Work out the finished part from the listing and answer in its coordinate system (mm). A direction names the side the tool comes from. Coordinates: 2 decimals unless noted, no trailing zeros. Order: outer loops, then holes, each group sorted by start corner. A loop starts at its lowest first (then second) coordinate and runs counter-clockwise, first axis right, second up. Notation, with made-up numbers: (57.25, 24.5) -> (99.25, 24.5) arc R14 ccw to (99.25, 29.5) -> close; hole circle Ø4 at (-20, 7.25). An arc over 180 degrees is marked (long way). Use one line per item in the form item = value.
from build123d import *

# Parameters (mm, degrees)
SKETCH_1_W          = 36
SKETCH_1_H          = 8
EXTRUDE_1_DEPTH     = 2
SKETCH_2_W          = 2
SKETCH_2_H          = 8
EXTRUDE_2_DEPTH     = 9
CUT_EXTRUDE_1_DEPTH = 21.518284529
SKETCH_4_R          = 1.6
CUT_EXTRUDE_2_DEPTH = 27.702059846
FILLET_1_R          = 1


with BuildPart() as part:
    # 草图1 → 凸台-拉伸1 (new body)
    with BuildSketch(Plane(origin=(0, 0, 0), x_dir=(1, 0, 0), z_dir=(0, 1, 0))):
        Rectangle(SKETCH_1_W, SKETCH_1_H)
        with BuildLine():
            Line((-15, 1.5), (-9, 1.5))
            ThreePointArc((-9, 1.5), (-7.5, 0), (-9, -1.5))
            Line((-9, -1.5), (-15, -1.5))
            ThreePointArc((-15, -1.5), (-16.5, 0), (-15, 1.5))
        make_face(mode=Mode.SUBTRACT)
        with BuildLine():
            Line((9, 1.5), (15, 1.5))
            ThreePointArc((15, 1.5), (16.5, 0), (15, -1.5))
            Line((15, -1.5), (9, -1.5))
            ThreePointArc((9, -1.5), (7.5, 0), (9, 1.5))
        make_face(mode=Mode.SUBTRACT)
    extrude(amount=EXTRUDE_1_DEPTH)

    # 草图2 → 凸台-拉伸2 (add)
    with BuildSketch(Plane(origin=(0, 2, 0), x_dir=(1, 0, 0), z_dir=(0, 1, 0))):
        with Locations((-5, 0)):
            Rectangle(SKETCH_2_W, SKETCH_2_H)
        with Locations((5, 0)):
            Rectangle(SKETCH_2_W, SKETCH_2_H)
    extrude(amount=EXTRUDE_2_DEPTH)

    # 草图3 → 切除-拉伸1 (cut, through all)
    with BuildSketch(Plane(origin=(0, 2, 0), x_dir=(1, 0, 0), z_dir=(0, 1, 0))):
        Polygon((2.5, -2.5), (4, -4), (-4, -4), (-2.5, -2.5), align=None)
        Polygon((-2.5, 2.5), (2.5, 2.5), (4, 4), (-4, 4), align=None)
    extrude(amount=-CUT_EXTRUDE_1_DEPTH, mode=Mode.SUBTRACT)

    # 草图4 → 切除-拉伸2 (cut, through all)
    with BuildSketch(Plane(origin=(6, 0, 0), x_dir=(0, 0, -1), z_dir=(1, 0, 0))):
        with Locations((0, 7)):
            Circle(SKETCH_4_R)
        with BuildLine():
            Line((-4, 11), (-4, 6.999999618))
            ThreePointArc((-4, 6.999999618), (-2.82842726, 9.82842699), (0, 11))
            Line((0, 11), (-4, 11))
        make_face()
        with BuildLine():
            ThreePointArc((0, 11), (2.828427125, 9.828427125), (4, 7))
            Line((4, 7), (4, 11))
            Line((4, 11), (0, 11))
        make_face()
    extrude(amount=-CUT_EXTRUDE_2_DEPTH, mode=Mode.SUBTRACT)

    # 圆角1
    fillet_1_edges = [part.edges().sort_by_distance(p)[0] for p in [
        (18, 1, 4),
        (-18, 1, 4),
        (-18, 1, -4),
        (18, 1, -4),
    ]]
    fillet(fillet_1_edges, radius=FILLET_1_R)


solid = part.part
(1) Section A-A on x = 13 is taken. Write down the section's boundary in (y, z), plus the area to 3 significant figures.
Data:
outline = (0, -4) -> (2, -4) -> (2, -1.5) -> (0, -1.5) -> close; (0, 1.5) -> (2, 1.5) -> (2, 4) -> (0, 4) -> close
area = 10.0 mm²
(2) Straight lines are drawn through the part: line 1 along X through (y, z) = (4.25, 1.25); line 2 along Z through (x, y) = (10, 1.5); line 3 along Y through (x, z) = (-5, 0). For each, find the intervals that lie inside material, in ascending order.
Data:
line_1 = -6 to -4, 4 to 6
line_2 = -4 to -1.5, 1.5 to 4
line_3 = 0 to 5.4, 8.6 to 11
(3) Section C-C on y = 7.5 is taken. Write down the section's boundary in (x, z).
Data:
outline = (-6, -3.97) -> (-4, -3.97) -> (-4, -1.52) -> (-6, -1.52) -> close; (-6, 1.52) -> (-4, 1.52) -> (-4, 3.97) -> (-6, 3.97) -> close; (4, -3.97) -> (6, -3.97) -> (6, -1.52) -> (4, -1.52) -> close; (4, 1.52) -> (6, 1.52) -> (6, 3.97) -> (4, 3.97) -> close
(4) Each of these flat-tipped pins is pushed along its axis until it touches: P1, Ø2.5, axis at x = 9.5, z = -0.5, coming from the +Y side; P2, Ø2.5, axis at y = 7, z = 0, coming from the -X side; P3, Ø4, axis at y = 5.5, z = 0.5, coming from the -X side; P4, Ø2.5, axis at y = 7.5, z = 0.5, coming from the +X side. Where does it stop, or does it pass through?
Data:
P1 = 2
P2 = through
P3 = -6
P4 = 6
(5) Section D-D on x = -6.5 is taken. Write down the section's boundary in (y, z), plus the area to 3 significant figures.
Data:
outline = (0, -4) -> (2, -4) -> (2, 4) -> (0, 4) -> close
area = 16.0 mm²
(6) The mould has two halves that part along X. Classify faces 4 (the cylindrical face through (-7.5, 1, 0)), 5 (the cylindrical face through (16.5, 1, 0)), 6 (the flat face through (-9, 1, 4)), 7 (the flat face through (6, 5, 1)): released by +X, released by -X, zero draft, split by the parting line, or undercut.
Data:
face_4 = undercut
face_5 = undercut
face_6 = zero draft
face_7 = released by +X
(7) Section B-B on y = 5 is taken. Write down the section's boundary in (x, z).
Data:
outline = (-6, -4) -> (-4, -4) -> (-4, 4) -> (-6, 4) -> close; (4, -4) -> (6, -4) -> (6, 4) -> (4, 4) -> close
(8) Which of the six approach directions +Z, -Z, +X, -X, +Y, -Y give full straight-line access (tool end or side, diameter ignored) to faces 1 (the flat face through (3, 1, 3)), 2 (the flat face through (0, 2, 0)), 3 (the flat face through (12, 1, -1.5))?
Data:
face_1 = +Z, +Y, -Y
face_2 = +Z, -Z, +Y
face_3 = +Y, -Y
